from build123d import *

# Parameters (mm, degrees)
SKETCH_1_W          = 178
SKETCH_1_H          = 70
EXTRUDE_1_DEPTH     = 4
SKETCH_2_R          = 13.25
SKETCH_2_R_2        = 2.075
SKETCH_2_R_3        = 1.575
SKETCH_2_W          = 4
SKETCH_2_H          = 20
CUT_EXTRUDE_1_DEPTH = 192.311264697


with BuildPart() as part:
    # 草图1 → 凸台-拉伸1 (new body)
    with BuildSketch(Plane.XY):
        with Locations((89, -35)):
            Rectangle(SKETCH_1_W, SKETCH_1_H)
    extrude(amount=EXTRUDE_1_DEPTH)

    # 草图2 → 切除-拉伸1 (cut, through all)
    with BuildSketch(Plane.XY.offset(4)):
        with Locations((89, -35)):
            Circle(SKETCH_2_R)
        with Locations((89, -17.5)):
            Circle(SKETCH_2_R_2)
        with Locations((106.5, -35)):
            Circle(SKETCH_2_R_2)
        with Locations((89, -52.5)):
            Circle(SKETCH_2_R_2)
        with Locations((71.5, -35)):
            Circle(SKETCH_2_R_2)
        with Locations((9, -5)):
            Circle(SKETCH_2_R_3)
        with Locations(Location((9, -65, 0), (0, 0, 180))):
            Circle(SKETCH_2_R_3)
        with Locations((169, -65)):
            Circle(SKETCH_2_R_3)
        with Locations(Location((169, -5, 0), (0, 0, 180))):
            Circle(SKETCH_2_R_3)
        Polygon((40.196152423, -11), (35, -14), (35, -20), (40.196152423, -23), (45.392304845, -20), (45.392304845, -14), align=None)
        with Locations((2, -10)):
            Rectangle(SKETCH_2_W, SKETCH_2_H)
        with Locations((176, -10)):
            Rectangle(SKETCH_2_W, SKETCH_2_H)
        with Locations((176, -60)):
            Rectangle(SKETCH_2_W, SKETCH_2_H)
        with Locations((2, -60)):
            Rectangle(SKETCH_2_W, SKETCH_2_H)
        Polygon((26.196152423, -23), (31.392304845, -20), (31.392304845, -14), (26.196152423, -11), (21, -14), (21, -20), align=None)
        Polygon((33.196152423, -35), (38.392304845, -32), (38.392304845, -26), (33.196152423, -23), (28, -26), (28, -32), align=None)
        Polygon((47.196152423, -23), (42, -26), (42, -32), (47.196152423, -35), (52.392304845, -32), (52.392304845, -26), align=None)
        Polygon((14, -26), (19.196152423, -23), (24.392304845, -26), (24.392304845, -32), (19.196152423, -35), (14, -32), align=None)
        Polygon((35, -44), (35, -38), (40.196152423, -35), (45.392304845, -38), (45.392304845, -44), (40.196152423, -47), align=None)
        Polygon((21, -38), (26.196152423, -35), (31.392304845, -38), (31.392304845, -44), (26.196152423, -47), (21, -44), align=None)
        Polygon((14, -50), (14, -56), (19.196152423, -59), (24.392304845, -56), (24.392304845, -50), (19.196152423, -47), align=None)
        Polygon((42, -56), (42, -50), (47.196152423, -47), (52.392304845, -50), (52.392304845, -56), (47.196152423, -59), align=None)
        Polygon((28, -50), (33.196152423, -47), (38.392304845, -50), (38.392304845, -56), (33.196152423, -59), (28, -56), align=None)
        Polygon((144.803847577, -47), (139.607695155, -50), (139.607695155, -56), (144.803847577, -59), (150, -56), (150, -50), align=None)
        Polygon((130.803847577, -59), (136, -56), (136, -50), (130.803847577, -47), (125.607695155, -50), (125.607695155, -56), align=None)
        Polygon((164, -56), (158.803847577, -59), (153.607695155, -56), (153.607695155, -50), (158.803847577, -47), (164, -50), align=None)
        Polygon((137.803847577, -47), (143, -44), (143, -38), (137.803847577, -35), (132.607695155, -38), (132.607695155, -44), align=None)
        Polygon((151.803847577, -35), (146.607695155, -38), (146.607695155, -44), (151.803847577, -47), (157, -44), (157, -38), align=None)
        Polygon((164, -32), (164, -26), (158.803847577, -23), (153.607695155, -26), (153.607695155, -32), (158.803847577, -35), align=None)
        Polygon((136, -26), (136, -32), (130.803847577, -35), (125.607695155, -32), (125.607695155, -26), (130.803847577, -23), align=None)
        Polygon((150, -32), (144.803847577, -35), (139.607695155, -32), (139.607695155, -26), (144.803847577, -23), (150, -26), align=None)
        Polygon((143, -14), (143, -20), (137.803847577, -23), (132.607695155, -20), (132.607695155, -14), (137.803847577, -11), align=None)
        Polygon((157, -20), (151.803847577, -23), (146.607695155, -20), (146.607695155, -14), (151.803847577, -11), (157, -14), align=None)
    extrude(amount=-CUT_EXTRUDE_1_DEPTH, mode=Mode.SUBTRACT)


solid = part.part
Could you check a few things on this model? Use its own coordinates, in mm. Give positions to 0.01 mm unless a question says otherwise; leave off trailing zeros. Order: outer loops, then holes, each group sorted by start corner. A loop starts at its lowest first (then second) coordinate and runs counter-clockwise, first axis right, second up. Notation, with made-up numbers: (86, 85) - (98, 85) arc R24 cw to (98, 109) - close; hole circle Ø4 at (40.5, 55.25). An arc over 180 degrees is marked (long way). Return JSON: item names as keys, results as strings. Group by question number.
Q1. Please list where these lines run through material, in increasing order: line 1 along X through (y, z) = (-65, 1.45) (3 decimals); line 2 along Y through (x, z) = (169, 2.9) (3 decimals); line 3 along X through (y, z) = (-38.5, 2.65). Write a range as [from, to].
Q2. Suppose I cut it at D-D, the plane y = -65. Please give me the cut outline in (x, z) (3 decimals), and give its area (3 significant figures).
Q3. Suppose I cut it at B-B, the plane x = 106.5. Please give me the cut outline in (y, z) (3 decimals).
Q4. Will these pins go through, and if not, where does the flat tip stop? pin 1 Ø1.2 at (x, z) = (177, 3) entering from +Y; pin 2 Ø6 at (x, y) = (27.5, -59) entering from -Z; pin 3 Ø2 at (y, z) = (-52, 2) entering from -X; pin 4 Ø3.5 at (x, y) = (71.5, -35) entering from +Z.
Q5. Suppose I cut it at C-C, the plane x = 9. Please give me the cut outline in (y, z) (3 decimals).
Q6. Thinking about a two-plate mould opening in X: for faces 1 (the face through (88, -50, 4)), 2 (the face through (164, -29, 2)), which applies, pulls with the +X half, pulls with the -X half, needs draft (parallel to the pull), parting line crosses it, or undercut?
Q7. Suppose I cut it at A-A, the plane y = -17.5. Please give me the cut outline in (x, z) (3 decimals).
Resolved:
{
 "1": {"line 1": "x = [4, 7.425], [10.575, 167.425], [170.575, 174]", "line 2": "y = [-70, -66.575], [-63.425, -6.575], [-3.425, 0]", "line 3": "x = [0, 21], [31.39, 35], [45.39, 76.22], [101.78, 132.61], [143, 146.61], [157, 178]"},
 "2": {"outline": "(4, 0) - (7.425, 0) - (7.425, 4) - (4, 4) - close; (10.575, 0) - (167.425, 0) - (167.425, 4) - (10.575, 4) - close; (170.575, 0) - (174, 0) - (174, 4) - (170.575, 4) - close", "area": "655 mm2"},
 "3": {"outline": "(-70, 0) - (-37.075, 0) - (-37.075, 4) - (-70, 4) - close; (-32.925, 0) - (0, 0) - (0, 4) - (-32.925, 4) - close"},
 "4": {"pin 1": "stops at y = -20", "pin 2": "stops at z = 0", "pin 3": "stops at x = 4", "pin 4": "passes through"},
 "5": {"outline": "(-70, 0) - (-66.575, 0) - (-66.575, 4) - (-70, 4) - close; (-63.425, 0) - (-6.575, 0) - (-6.575, 4) - (-63.425, 4) - close; (-3.425, 0) - (0, 0) - (0, 4) - (-3.425, 4) - close"},
 "6": {"face 1": "needs draft", "face 2": "undercut"},
 "7": {"outline": "(4, 0) - (21, 0) - (21, 4) - (4, 4) - close; (31.392, 0) - (35, 0) - (35, 4) - (31.392, 4) - close; (45.392, 0) - (86.925, 0) - (86.925, 4) - (45.392, 4) - close; (91.075, 0) - (132.608, 0) - (132.608, 4) - (91.075, 4) - close; (143, 0) - (146.608, 0) - (146.608, 4) - (143, 4) - close; (157, 0) - (174, 0) - (174, 4) - (157, 4) - close"}
}
